Can you work these out from the model? Positions are in its coordinate system, mm. A direction names the side the tool comes from. Coordinates: 2 decimals unless noted, no trailing zeros. Order: outer loops, then holes, each group sorted by start corner. A loop starts at its lowest first (then second) coordinate and runs counter-clockwise, first axis right, second up. Notation, with made-up numbers: (87, -39.75) - (135, -39.75) arc R29 ccw to (135, -12.75) - close; hole circle Ø10 at (84.25, 5). An arc over 180 degrees is marked (long way). Return JSON: item names as keys, results as strings. Group by question number.
1) Imagine slicing it at A-A (x = 17). Write out the boundary of the cut face in (y, z), and give its area (3 significant figures).
2) Which directions (+Z, -Z, +X, -X, +Y, -Y) give clear straight access to the entire face, cutting with the end or side of a thin tool? Please do faces 1 (the face through (0, 3, 0)), 2 (the face through (-15, 3, 0)), 3 (the face through (7, 9, 0)).
3) Imagine slicing it at D-D (y = 13). Write out the boundary of the cut face in (x, z), and give its area (3 significant figures).
4) If we mould it in two halves opening along Y, with no side actions, what happens to faces 4 (the face through (-18.6, 1.48, -0.07)), 5 (the face through (5, 17, 0)), 6 (the face through (5.479, 14.586, 0.208))? For each: pulls with the +Y half, pulls with the -Y half, needs draft (parallel to the pull), parting line crosses it, or undercut.
5) For pin 1 Ø5 at (y, z) = (8.5, 2) entering from +X; pin 2 Ø2.5 at (x, z) = (1.5, -0.5) entering from +Y; pin 3 Ø4 at (y, z) = (13, 0) entering from -X; pin 4 Ø3 at (x, z) = (-17, 0) entering from +Y, each with a flat end and sliding along its axis, tell me the tip position at first contact or that it passes through.
6) Imagine slicing it at B-B (z = 0). Write out the boundary of the cut face in (x, y), and give its area (3 significant figures).
7) Imagine slicing it at C-C (y = 7.75). Write out the boundary of the cut face in (x, z), and give its area (3 significant figures).
8) If I drill on line 1 along X through (y, z) = (2.4, 0); line 2 along X through (y, z) = (3.25, -1.5); line 3 along Y through (x, z) = (4.9, 0), over which ranges is the centre line in solid material (lowest first)?
```python
from build123d import *

# Parameters (mm, degrees)
SKETCH_1_W      = 44
SKETCH_1_H      = 10
SKETCH_1_R      = 1.6
EXTRUDE_1_DEPTH = 3
SKETCH_2_R      = 4
SKETCH_2_R_2    = 1.6
EXTRUDE_2_DEPTH = 3


with BuildPart() as part:
    # 草图1 → 凸台-拉伸1 (new body)
    with BuildSketch(Plane(origin=(0, 0, 0), x_dir=(1, 0, 0), z_dir=(0, 1, 0))):
        Rectangle(SKETCH_1_W, SKETCH_1_H)
        with Locations((17, 0)):
            Circle(SKETCH_1_R, mode=Mode.SUBTRACT)
        with Locations((-17, 0)):
            Circle(SKETCH_1_R, mode=Mode.SUBTRACT)
    extrude(amount=EXTRUDE_1_DEPTH)

    # 草图2 → 凸台-拉伸2 (add)
    with BuildSketch(Plane(origin=(4, 0, 0), x_dir=(0, 0, -1), z_dir=(1, 0, 0))):
        with BuildLine():
            Line((-5, 3), (5, 3))
            Line((5, 3), (3.980898083, 13.390449041))
            ThreePointArc((3.980898083, 13.390449041), (3.995221667, 13.195458012), (4, 13))
            ThreePointArc((4, 13), (-0.195458012, 9.004778333), (-3.980898083, 13.390449041))
            Line((-3.980898083, 13.390449041), (-5, 3))
        make_face()
        with Locations((0, 13)):
            Circle(SKETCH_2_R)
        with Locations((0, 13)):
            Circle(SKETCH_2_R_2, mode=Mode.SUBTRACT)
    extrude_2 = extrude(amount=EXTRUDE_2_DEPTH)

    # 镜向1: 凸台-拉伸2 across plane
    add(extrude_2.mirror(Plane(origin=(0, 0, 0), x_dir=(0, 0, 1), z_dir=(1, 0, 0))))


solid = part.part
```
Calculated:
{
 "1": {"outline": "(0, -5) - (3, -5) - (3, -1.6) - (0, -1.6) - close; (0, 1.6) - (3, 1.6) - (3, 5) - (0, 5) - close", "area": "20.4 mm2"},
 "2": {"face 1": "+Z, -Z, +Y", "face 2": "+Z, -Z, -X, +Y", "face 3": "+Z, -Z, +X, +Y"},
 "3": {"outline": "(-7, -4.02) - (-4, -4.02) - (-4, -1.6) - (-7, -1.6) - close; (-7, 1.6) - (-4, 1.6) - (-4, 4.02) - (-7, 4.02) - close; (4, -4.02) - (7, -4.02) - (7, -1.6) - (4, -1.6) - close; (4, 1.6) - (7, 1.6) - (7, 4.02) - (4, 4.02) - close", "area": "29.0 mm2"},
 "4": {"face 4": "needs draft", "face 5": "pulls with the +Y half", "face 6": "undercut"},
 "5": {"pin 1": "x = 7", "pin 2": "y = 3", "pin 3": "x = -7", "pin 4": "through"},
 "6": {"outline": "(-22, 0) - (-18.6, 0) - (-18.6, 3) - (-22, 3) - close; (-15.4, 0) - (15.4, 0) - (15.4, 3) - (7, 3) - (7, 11.4) - (4, 11.4) - (4, 3) - (-4, 3) - (-4, 11.4) - (-7, 11.4) - (-7, 3) - (-15.4, 3) - close; (-7, 14.6) - (-4, 14.6) - (-4, 17) - (-7, 17) - close; (4, 14.6) - (7, 14.6) - (7, 17) - (4, 17) - close; (18.6, 0) - (22, 0) - (22, 3) - (18.6, 3) - close", "area": "178 mm2"},
 "7": {"outline": "(-7, -4.53) - (-4, -4.53) - (-4, 4.53) - (-7, 4.53) - close; (4, -4.53) - (7, -4.53) - (7, 4.53) - (4, 4.53) - close", "area": "54.4 mm2"},
 "8": {"line 1": "-22 to -18.6, -15.4 to 15.4, 18.6 to 22", "line 2": "-7 to -4, 4 to 7", "line 3": "0 to 11.4, 14.6 to 17"}
}
